Source: CAD feature listing. Evaluate the final solid. Frame: model axes, mm. Round coordinates to 2 decimals unless told otherwise and drop trailing zeros. Loops run counter-clockwise (first coordinate to the right, second up) from the corner with the lowest first, then second, coordinate; pieces in that order, holes last. Notation, with made-up numbers: M -7.5,82 L 10.5,82 A9 cw 10.5,86 Z; hole C 37,64 d10. An arc over 180 degrees is marked long. Write each question's results on one line, items separated by ' | '. Start each with the question number.
1. Contact query for flat-ended pins moving along their axis: pin 1 Ø3 at (x, z) = (-20.45, -11.27) entering from -Y; pin 2 Ø2 at (x, z) = (-125, -17) entering from -Y; pin 3 Ø5 at (x, y) = (-144, 10) entering from -Z (3 decimals); pin 4 Ø6 at (x, z) = (-199.2, -11.27) entering from +Y (3 decimals). Output: stop coordinate, or through.
2. Ray query, line 1 (Z direction, x = -91.95, y = 1.7); line 2 (Z direction, x = -104.5, y = 3.75) (3 decimals); line 3 (Y direction, x = -124.5, z = -15.75) (3 decimals). Return the intervals inside material, ascending.
3. Section A-A on y = 14. Output: boundary loops of the cut face in (x, z) (3 decimals), and give its area (3 significant figures).
from build123d import *

# Parameters (mm, degrees)
BOSS_EXTRUDE1_DEPTH = 468
SKETCH2_R           = 2.38125
CUT_EXTRUDE1_DEPTH  = 3.175


with BuildPart() as part:
    # Sketch1 → Boss-Extrude1 (new body)
    with BuildSketch(Plane(origin=(0, 0, 0), x_dir=(0, 0, -1), z_dir=(1, 0, 0))):
        Polygon((0, 0), (0, 19.05), (3.175, 19.05), (3.175, 3.175), (19.05, 3.175), (19.05, 0), align=None)
    extrude(amount=-BOSS_EXTRUDE1_DEPTH)

    # Sketch2 → Cut-Extrude1 (cut)
    with BuildSketch(Plane(origin=(0, 3.175, 0), x_dir=(1, 0, 0), z_dir=(0, 1, 0))):
        with Locations((-20.45, 11.273546723)):
            Circle(SKETCH2_R)
        with Locations((-56.2, 11.273546723)):
            Circle(SKETCH2_R)
        with Locations((-91.95, 11.273546723)):
            Circle(SKETCH2_R)
        with Locations((-127.7, 11.273546723)):
            Circle(SKETCH2_R)
        with Locations((-163.45, 11.273546723)):
            Circle(SKETCH2_R)
        with Locations((-199.2, 11.273546723)):
            Circle(SKETCH2_R)
        with Locations((-234.95, 11.273546723)):
            Circle(SKETCH2_R)
        with Locations((-270.7, 11.273546723)):
            Circle(SKETCH2_R)
        with Locations((-306.45, 11.273546723)):
            Circle(SKETCH2_R)
        with Locations((-342.2, 11.273546723)):
            Circle(SKETCH2_R)
        with Locations((-377.95, 11.273546723)):
            Circle(SKETCH2_R)
        with Locations((-413.7, 11.273546723)):
            Circle(SKETCH2_R)
        with Locations((-449.45, 11.273546723)):
            Circle(SKETCH2_R)
    extrude(amount=-CUT_EXTRUDE1_DEPTH, mode=Mode.SUBTRACT)


solid = part.part
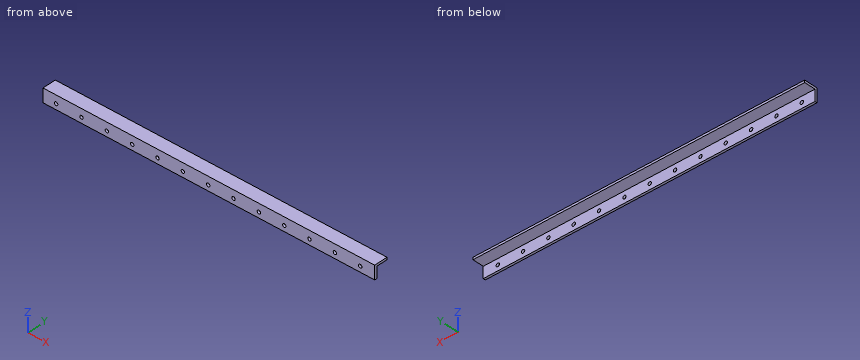
Taken from the geometry:
1) pin 1: through | pin 2: y = 0 | pin 3: z = -3.175 | pin 4: y = 3.175
2) line 1: -19.05 to -13.65, -8.89 to 0 | line 2: -3.175 to 0 | line 3: 0 to 3.175
3) outline: M -468,-3.175 L 0,-3.175 L 0,0 L -468,0 Z | area: 1,490 mm^2
